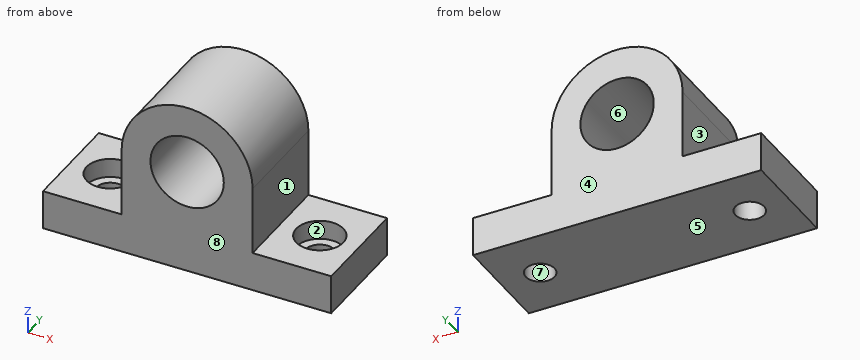
```python
from build123d import *

# Parameters (mm, degrees)
F0_R     = 14
F1_DEPTH = 40
F2_R     = 9
F3_DEPTH = 7.3
F4_R     = 5.5
F5_R     = 5.5
F6_DEPTH = 25


with BuildPart() as f1:
    # F0 (on Front) → F1 (new body)
    with BuildSketch(Plane.XZ):
        with BuildLine():
            Line((-15.140404, -10.733506), (-45.140404, -10.733506))
            Line((-45.140404, -10.733506), (-45.140404, -25.733506))
            Line((-45.140404, -25.733506), (64.859596, -25.733506))
            Line((64.859596, -25.733506), (64.859596, -10.733506))
            Line((64.859596, -10.733506), (34.859596, -10.733506))
            Line((34.859596, -10.733506), (34.859596, 15.266494))
            ThreePointArc((34.859596, 15.266494), (9.859596, 40.266494), (-15.140404, 15.266494))
            Line((-15.140404, 15.266494), (-15.140404, -10.733506))
        make_face()
        with Locations((9.859596, 14.266494)):
            Circle(F0_R, mode=Mode.SUBTRACT)
    extrude(amount=F1_DEPTH)

    # F2 (on face) → F3 (cut)
    with BuildSketch(Plane.XY.offset(-10.733506)):
        with Locations((-30.140404, -20)):
            Circle(F2_R)
        with Locations((49.859596, -20)):
            Circle(F2_R)
    extrude(amount=-F3_DEPTH, mode=Mode.SUBTRACT)

    # F4 (on face) + F5 (on face) → F6 (cut)
    with BuildSketch(Plane.XY.offset(-18.033506)):
        with Locations((-30.140404, -20)):
            Circle(F4_R)
    with BuildSketch(Plane.XY.offset(-18.033506)):
        with Locations((49.859596, -20)):
            Circle(F5_R)
    extrude(amount=-F6_DEPTH, mode=Mode.SUBTRACT)


solid = f1.part
```
For this review, take the finished solid that the model builds, in its own axes (mm). Face numbers are marked on the shaded views. A direction names the side the tool comes from. Coordinates: 2 decimals unless noted, no trailing zeros. Loops run counter-clockwise (first coordinate to the right, second up) from the corner with the lowest first, then second, coordinate; pieces in that order, holes last. Notation, with made-up numbers: (-28, 64) -> (-7, 64) arc R17 cw to (-7, 80) -> close; hole circle Ø11 at (42, -34.75). An arc over 180 degrees is marked (long way). Return JSON: item names as keys, results as strings. Group by question number.
(1) Consider section B-B, the plane x = -28. Give the boundary of the cut face in (y, z), plus the area to 3 significant figures.
(2) Consider section C-C, the plane y = -20. Give the boundary of the cut face in (x, z), plus the area to 3 significant figures.
(3) Consider section D-D, the plane z = 18. Give the boundary of the cut face in (x, y), plus the area to 3 significant figures.
(4) Consider section A-A, the plane z = -14. Give the boundary of the cut face in (x, y).
(5) Tool access review of the marked faces 1, 2, 3, 4 and 5: name each direction out of +Z, -Z, +X, -X, +Y, -Y from which nothing blocks a thin tool from reaching the whole face with its end or side.
(6) Mouldability with a two-part tool opening along Y and no side actions: class the marked faces 6, 7 and 8 as pulls with the +Y half, pulls with the -Y half, needs draft (parallel to the pull), parting line crosses it, or undercut.
(7) To check wall thickness, follow L1, parallel to X at y = -30.5, z = 14; L2, parallel to Z at x = 53, y = -12; L3, parallel to Z at x = 36, y = -24. State the ranges of each line that lie inside material, in increasing order.
(8) For pin 1 Ø13 at (y, z) = (-23.5, -4) entering from -X; pin 2 Ø4 at (y, z) = (-21, -7) entering from +X; pin 3 Ø25 at (x, z) = (9.86, 14.27) entering from -Y; pin 4 Ø20 at (x, y) = (-30, -22.5) entering from +Z, all flat-tipped, find the tip position at first contact; note any pin that passes through.
Results below:
{
 "1": {"outline": "(-40, -25.73) -> (-25.07, -25.73) -> (-25.07, -18.03) -> (-28.74, -18.03) -> (-28.74, -10.73) -> (-40, -10.73) -> close; (-14.93, -25.73) -> (0, -25.73) -> (0, -10.73) -> (-11.26, -10.73) -> (-11.26, -18.03) -> (-14.93, -18.03) -> close", "area": "394 mm2"},
 "2": {"outline": "(-45.14, -25.73) -> (-35.64, -25.73) -> (-35.64, -18.03) -> (-39.14, -18.03) -> (-39.14, -10.73) -> (-45.14, -10.73) -> close; (-24.64, -25.73) -> (44.36, -25.73) -> (44.36, -18.03) -> (40.86, -18.03) -> (40.86, -10.73) -> (34.86, -10.73) -> (34.86, 15.27) arc R25 ccw to (-15.14, 15.27) -> (-15.14, -10.73) -> (-21.14, -10.73) -> (-21.14, -18.03) -> (-24.64, -18.03) -> close; (55.36, -25.73) -> (64.86, -25.73) -> (64.86, -10.73) -> (58.86, -10.73) -> (58.86, -18.03) -> (55.36, -18.03) -> close; hole circle Ø28 at (9.86, 14.27)", "area": "2,880 mm2"},
 "3": {"outline": "(-14.99, -40) -> (-3.63, -40) -> (-3.63, 0) -> (-14.99, 0) -> close; (23.35, -40) -> (34.71, -40) -> (34.71, 0) -> (23.35, 0) -> close", "area": "909 mm2"},
 "4": {"outline": "(-45.14, -40) -> (64.86, -40) -> (64.86, 0) -> (-45.14, 0) -> close; hole circle Ø18 at (-30.14, -20); hole circle Ø18 at (49.86, -20)"},
 "5": {"face 1": "+Z, +X, +Y, -Y", "face 2": "+Z", "face 3": "+Z, -X, +Y, -Y", "face 4": "+Z, -Z, +X, -X, +Y", "face 5": "-Z, +X, -X, +Y, -Y"},
 "6": {"face 6": "needs draft", "face 7": "undercut", "face 8": "pulls with the -Y half"},
 "7": {"L1": "x = -15.14 to -4.14, 23.86 to 34.86", "L2": "z = -25.73 to -18.03", "L3": "z = -25.73 to -10.73"},
 "8": {"pin 1": "stops at x = -15.14", "pin 2": "stops at x = 34.86", "pin 3": "passes through", "pin 4": "stops at z = -10.73"}
}
